Build history of the part. All positions in model axes, mm. A direction names the side the tool comes from. Coordinates: 2 decimals unless noted, no trailing zeros. Write each loop counter-clockwise with the first axis right and the second up, starting at its lowest first coordinate (ties: lowest second). Pieces come first, ordered by that corner, then holes.
Autodesk Fusion 360 part; units mm, degrees
sketch "Sketch1" plane through (0, 0, 0) normal (0, 0, 1) x (1, 0, 0)
  circle A0 centre (0, 0) radius 10
extrude "Extrude1" add sketch "Sketch1" along normal blind 6.5
sketch "Sketch2" plane through (0, 0, 0) normal (0, 0, -1) x (1, 0, 0)
  circle A0 centre (0, 0) radius 10
  line L0 (0, 2.5) -> (30, 2.5)
  line L1 (30, 2.5) -> (30, -2.5)
  line L2 (30, -2.5) -> (0, -2.5)
  line L3 (0, -2.5) -> (0, 2.5)
  line L4 (0, 2.5) -> (30, -2.5) construction
  line L5 (30, 2.5) -> (0, -2.5) construction
  line L6 (15, 0) -> (0, 0) construction
  point P0 (15, 0)
  dimension "d19" = 5
  dimension "d20" = 30
extrude "Extrude2" add sketch "Sketch2" against normal up to surface (6.5 mm away) contours A0 L0 L1 L2
hole "Hole1" at (0, 0, 6.5) direction (0, 0, -1) diameter 3 end through all
fillet "Fillet1" radius 2.5 2 edges at (30, -2.5, 3.25) (30, 2.5, 3.25)
hole "Hole2" at (27.5, 0, 6.5) direction (0, 0, -1) diameter 2.5 end through all
sketch "Sketch4" plane through (0, 0, 0) normal (0, 0, -1) x (1, 0, 0)
  circle A0 centre (27.5, 0) radius 1.25
  circle A1 centre (0, 0) radius 1.5
  arc A2 (27.5, -2.5) -> (27.5, 2.5) centre (27.5, 0) ccw
  line L0 (27.5, 2.5) -> (9.6825, 2.5)
  arc A3 (9.6825, 2.5) -> (9.6825, -2.5) centre (0, 0) ccw
  line L1 (9.6825, -2.5) -> (27.5, -2.5)
  line L2 (1.5, 5.546) -> (23.5, 5.546)
  line L3 (23.5, 5.546) -> (23.5, -5.546)
  line L4 (23.5, -5.546) -> (1.5, -5.546)
  line L5 (1.5, -5.546) -> (1.5, 5.546)
  line L6 (1.5, 5.546) -> (23.5, -5.546) construction
  line L7 (23.5, 5.546) -> (1.5, -5.546) construction
  line L8 (12.5, 0) -> (23.5, 0) construction
  point P0 (12.5, 0)
  dimension "d35" = 4
extrude "Extrude4" add sketch "Sketch4" against normal up to surface (6.5 mm away) contours A3 L1 L3 L4 | L0 A3 L2 L3
sketch "Sketch6" plane through (0, 0, 6.5) normal (0, 0, 1) x (-1, 0, 0)
  line L0 (-23.5, 5.546) -> (-23.5, 2.5)
  line L1 (-23.5, 2.5) -> (-27.5, 2.5)
  arc A0 (-27.5, 2.5) -> (-27.5, -2.5) centre (-27.5, 0) ccw
  line L2 (-27.5, -2.5) -> (-23.5, -2.5)
  line L3 (-23.5, -2.5) -> (-23.5, -5.546)
  line L4 (-23.5, -5.546) -> (-8.3212, -5.546)
  arc A1 (-8.3212, -5.546) -> (-8.3212, 5.546) centre (0, 0) ccw
  line L5 (-8.3212, 5.546) -> (-23.5, 5.546)
  circle A2 centre (-27.5, 0) radius 1.25
  circle A3 centre (0, 0) radius 1.5
  circle A4 centre (-21, 0) radius 1
  dimension "d36" = 2.5
fillet "Fillet2" radius 1 4 edges at (23.5, 5.546, 3.25) (23.5, -5.546, 3.25) (23.5, 2.5, 3.25) (23.5, -2.5, 3.25)
hole "Hole4" at (21, 0, 6.5) direction (0, 0, -1) diameter 3 end through all
1. 3-axis set-ups, long thin cutter, end or side, ignore diameter. For faces 1 (the face through (-10, 0, 3)), 2 (the face through (16, 5.546, 3)), 3 (the face through (15, -5.546, 3)): which of +Z, -Z, +X, -X, +Y, -Y reach the whole face in a straight line?
Computed values:
face 1: +Z, -Z
face 2: +Z, -Z, +X, +Y
face 3: +Z, -Z, +X, -Y
2. Saw through at D-D on x = 21.5. List the corners of the cut face in (y, z).
Computed values:
outline: (-5.55, 0) - (-1.41, 0) - (-1.41, 6.5) - (-5.55, 6.5) - close; (1.41, 0) - (5.55, 0) - (5.55, 6.5) - (1.41, 6.5) - close
3. Saw through at B-B on y = -0.5. List the corners of the cut face in (x, z).
Computed values:
outline: (-9.99, 0) - (-1.41, 0) - (-1.41, 6.5) - (-9.99, 6.5) - close; (1.41, 0) - (19.59, 0) - (19.59, 6.5) - (1.41, 6.5) - close; (22.41, 0) - (26.35, 0) - (26.35, 6.5) - (22.41, 6.5) - close; (28.65, 0) - (29.95, 0) - (29.95, 6.5) - (28.65, 6.5) - close
4. Saw through at C-C on z = 4.5. State how many separate pieces and enclosed holes the cut face has, plus the area to 3 significant figures.
Computed values:
separate pieces: 1
enclosed holes: 3
area: 481 mm2
5. Flat gauge pins, fed straight in: pin 1 (3 mm diameter, centred on y = -4.5, z = 2.5, fed in from -X); pin 2 (0.9 mm diameter, centred on x = 26, z = 2.5, fed in from -Y); pin 3 (1.8 mm diameter, centred on x = 0, y = 0, fed in from -Z); pin 4 (1.5 mm diameter, centred on y = 1.5, z = 1.5, fed in from -X). Where does each tip first touch, or does it go through?
Computed values:
pin 1: stops at x = -9.54
pin 2: stops at y = -2.5
pin 3: passes through
pin 4: stops at x = -9.97
6. Mould opens along Y. For faces 4 (the face through (23.801, -2.785, 3.296)), 5 (the face through (23.21, 5.25, 3.3)), 6 (the face through (19.513, 0.195, 3.204)), 7 (the face through (-0.07, 1.5, 3.2)) say: +Y half, -Y half, draft (parallel to the pull), parting line (faces both ways), or undercut.
Computed values:
face 4: -Y half
face 5: +Y half
face 6: undercut
face 7: undercut
7. Probe line 1 along X through (y, z) = (0, 1.5); line 2 along X through (y, z) = (-0.5, 0.75); line 3 along Y through (x, z) = (21, 5). List the from-to ranges inside material, lowest first.
Computed values:
line 1: x = -10 to -1.5, 1.5 to 19.5, 22.5 to 26.25, 28.75 to 30
line 2: x = -9.99 to -1.41, 1.41 to 19.59, 22.41 to 26.35, 28.65 to 29.95
line 3: y = -5.55 to -1.5, 1.5 to 5.55
8. Saw through at A-A on x = 0. List the corners of the cut face in (y, z).
Computed values:
outline: (-10, 0) - (-1.5, 0) - (-1.5, 6.5) - (-10, 6.5) - close; (1.5, 0) - (10, 0) - (10, 6.5) - (1.5, 6.5) - close
